For this review, use the dimensioned drawing (mm, ordinates from the lowest corner) and the shaded views. Coordinates: 2 decimals unless noted, no trailing zeros. Write each loop counter-clockwise with the first axis right and the second up, starting at its lowest first coordinate (ties: lowest second). Pieces come first, ordered by that corner, then holes. Notation, with made-up numbers: M 34,51.5 L 39,51.5 A24 cw 39,73.5 Z; hole C 17.5,69.5 d11. An arc over 180 degrees is marked long. Return JSON: item names as keys, results as strings.
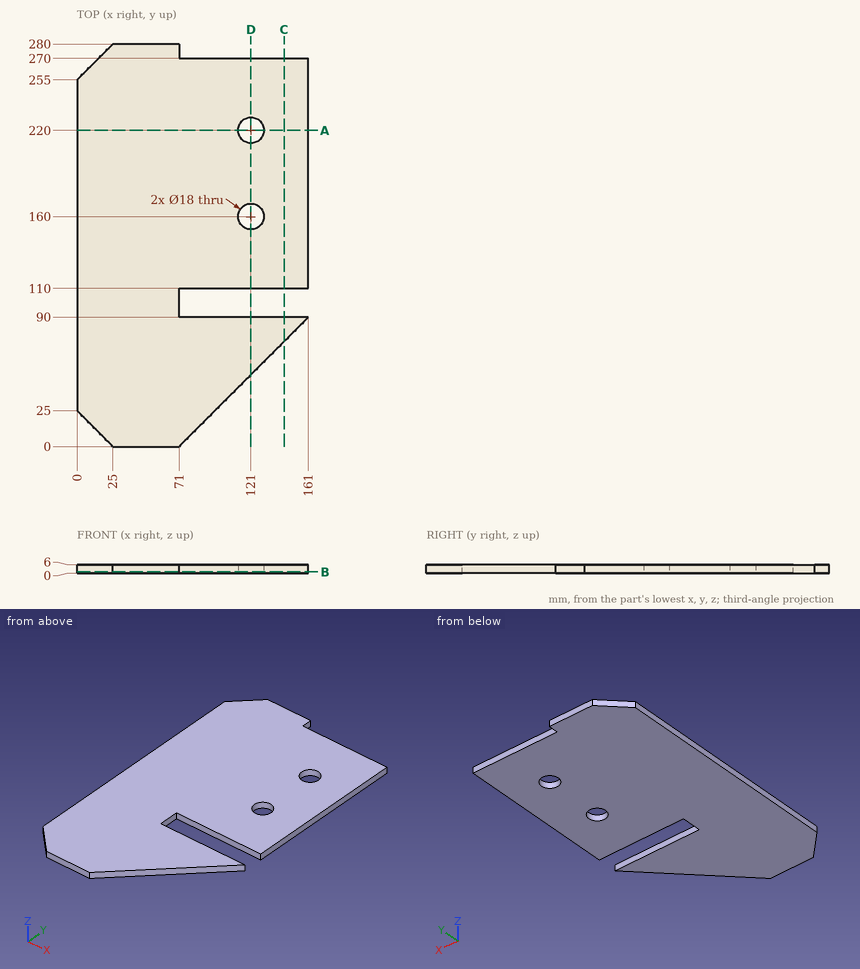
1. Wall thickness on L1, parallel to Y at x = 121, z = 4.2; L2, parallel to X at y = 220, z = 3.65; L3, parallel to Y at x = 124.5, z = 0.65: over which ranges is each line inside the solid? List them lowest first. Write a range as from..to.
Checks:
{"L1": "50..90, 110..151, 169..211, 229..270", "L2": "0..112, 130..161", "L3": "53.5..90, 110..151.71, 168.29..211.71, 228.29..270"}
2. We need section B-B (z = 0.9). State the section outline as (x, y) points, plus the area to 3 significant figures.
Checks:
{"outline": "M 0,25 L 25,0 L 71,0 L 161,90 L 71,90 L 71,110 L 161,110 L 161,270 L 71,270 L 71,280 L 25,280 L 0,255 Z; hole C 121,160 d18; hole C 121,220 d18", "area": "37,200 mm2"}
3. Clearance check with a flat-ended pin moving along its axis: pin 1 Ø16 at (x, y) = (121, 220) entering from +Z. State where the tip first meets the part, or that it passes through.
Checks:
{"pin 1": "through"}
4. We need section C-C (x = 144). State the section outline as (y, z) points, plus the area to 3 significant figures.
Checks:
{"outline": "M 73,0 L 90,0 L 90,6 L 73,6 Z; M 110,0 L 270,0 L 270,6 L 110,6 Z", "area": "1,060 mm2"}
5. We need section D-D (x = 121). State the section outline as (y, z) points.
Checks:
{"outline": "M 50,0 L 90,0 L 90,6 L 50,6 Z; M 110,0 L 151,0 L 151,6 L 110,6 Z; M 169,0 L 211,0 L 211,6 L 169,6 Z; M 229,0 L 270,0 L 270,6 L 229,6 Z"}
6. We need section A-A (y = 220). State the section outline as (x, z) points, plus the area to 3 significant figures.
Checks:
{"outline": "M 0,0 L 112,0 L 112,6 L 0,6 Z; M 130,0 L 161,0 L 161,6 L 130,6 Z", "area": "858 mm2"}
